Autodesk Inventor part; units mm, degrees
ref_plane "YZ Plane" through (0, 0, 0) normal (1, 0, 0) x (0, 1, 0)
ref_plane "XZ Plane" through (0, 0, 0) normal (0, 1, 0) x (-1, 0, 0)
ref_plane "XY Plane" through (0, 0, 0) normal (0, 0, 1) x (1, 0, 0)
sketch "Sketch1" plane through (0, 0, 0) normal (0, 0, 1) x (1, 0, 0)
  line L0 (0, 4) -> (0, 0)
  line L1 (0, 0) -> (125, 0)
  line L2 (125, 0) -> (125, 23.5)
  line L3 (57, 23.5) -> (0, 4)
  line L4 (81, 23.5) -> (81, 14.5)
  line L5 (81, 14.5) -> (92, 14.5)
  line L6 (92, 14.5) -> (92, 23.5)
  line L7 (125, 23.5) -> (92, 23.5)
  line L8 (81, 23.5) -> (57, 23.5)
  circle A0 centre (99.5, 19) radius 2.25
  circle A1 centre (119.5, 19) radius 2.25
  circle A2 centre (28.2, 6) radius 2.25
  circle A3 centre (28.2, 6) radius 4.5 construction
  point P0 (92, 19)
  dimension "d0" = 4
  dimension "d1" = 125
  dimension "d2" = 9
  dimension "d3" = 11
  dimension "d4" = 33
  dimension "d5" = 24
  dimension "d6" = 23.5
  dimension "d7" = 4.5
  dimension "d8" = 4.5
  dimension "d9" = 5.5
  dimension "d10" = 20
  dimension "d11" = 4.5
  dimension "d12" = 9
  dimension "d13" = 6
  dimension "d14" = 28.2
extrude "Extrusion1" add sketch "Sketch1" along normal blind 6.5
sketch "Sketch2" plane through (0, 0, 6.5) normal (0, 0, 1) x (1, 0, 0)
  line L0 (0, 0) -> (125, 0)
  line L1 (125, 23.5) -> (92, 23.5)
  line L2 (17, 0) -> (25, 0)
  line L3 (25, 0) -> (25, -4.5)
  line L4 (23, -6.5) -> (19, -6.5)
  line L5 (17, -4.5) -> (17, 0)
  line L6 (96, 0) -> (104, 0)
  line L7 (104, 0) -> (104, -19)
  line L8 (102, -21) -> (98, -21)
  line L9 (96, -19) -> (96, 0)
  line L10 (68, 0) -> (76, 0)
  line L11 (76, 0) -> (76, -19)
  line L12 (74, -21) -> (70, -21)
  line L13 (68, -19) -> (68, 0)
  line L14 (92, 23.5) -> (100, 23.5)
  line L15 (100, 23.5) -> (100, 29.5)
  line L16 (98, 31.5) -> (94, 31.5)
  line L17 (92, 29.5) -> (92, 23.5)
  arc A0 (17, -4.5) -> (19, -6.5) centre (19, -4.5) ccw
  arc A1 (23, -6.5) -> (25, -4.5) centre (23, -4.5) ccw
  arc A2 (96, -19) -> (98, -21) centre (98, -19) ccw
  arc A3 (102, -21) -> (104, -19) centre (102, -19) ccw
  arc A4 (68, -19) -> (70, -21) centre (70, -19) ccw
  arc A5 (74, -21) -> (76, -19) centre (74, -19) ccw
  arc A6 (94, 31.5) -> (92, 29.5) centre (94, 29.5) ccw
  arc A7 (100, 29.5) -> (98, 31.5) centre (98, 29.5) ccw
  line L18 (92, 23.5) -> (92, 14.5)
  dimension "d17" = 2
  dimension "d18" = 17
  dimension "d20" = 8
  dimension "d21" = 8
  dimension "d22" = 8
  dimension "d24" = 6.5
  dimension "d25" = 43
  dimension "d26" = 20
  dimension "d29" = 8
  dimension "d40" = 8
  dimension "d41" = 2
  dimension "d42" = 2
  dimension "d45" = 21
sketch "Sketch3" plane through (0, 0, 6.5) normal (0, 0, 1) x (1, 0, 0)
  circle A0 centre (119.5, 19) radius 2.25
  circle A1 centre (109.5, 19.599) radius 2.75
  circle A2 centre (86.5, 19.599) radius 7.5 construction
  dimension "d35" = 5.5
  dimension "d36" = 15
  dimension "d37" = 10
extrude "Extrusion3" cut sketch "Sketch3" against normal blind 6.5 contours A1
extrude "Extrusion4" add sketch "Sketch2" against normal blind 6.5
properties part number "x_motor_upper_nut_stop" material "Plywood, Finish"
Verification items for the finished model (mm, model axes). A direction names the side the tool comes from. Round coordinates to 2 decimals unless told otherwise and drop trailing zeros. Write each loop counter-clockwise with the first axis right and the second up, starting at its lowest first coordinate (ties: lowest second). Pieces come first, ordered by that corner, then holes.
1. Section check C-C on y = 25. Enter the section's corners in (x, z), plus the area to 3 significant figures.
2. Gauge pin test, flat ends, axial feed: P1, Ø3, axis at y = -13, z = 2.5, coming from the +X side; P2, Ø3.5, axis at y = -3, z = 2.5, coming from the -X side; P3, Ø3, axis at x = 116.5, z = 4.5, coming from the +Y side; P4, Ø2, axis at x = 97, z = 1, coming from the -Y side. Record the tip position at first contact, or that the pin passes through.
3. Section check A-A on x = 119.5. Enter the section's corners in (y, z).
4. Draft check along Y on faces 6 (the flat face through (104, -9, 3)), 7 (the cylindrical face through (107.318, 17.926, 3.296)), 8 (the flat face through (28.899, 13.887, 3.204)), 9 (the flat face through (21, -6.5, 3)). Enter one of: +Y half, -Y half, draft (parallel to the pull), parting line (faces both ways), or undercut.
5. Section check B-B on y = 6. Enter the section's corners in (x, z), plus the area to 3 significant figures.
6. Section check D-D on x = 62. Enter the section's corners in (y, z).
7. Access from +Z, -Z, +X, -X, +Y, -Y to the whole of each face (thin tool, end or side, straight path). Record for faces 1 (the flat face through (114, 0, 3)), 2 (the flat face through (100, 26, 3)), 3 (the flat face through (69, 23.5, 3)), 4 (the flat face through (25, -2, 3)), 5 (the flat face through (8, 0, 3)).
8. Scan lines: L1, parallel to X at y = -1.5, z = 4; L2, parallel to Y at x = 90, z = 6; L3, parallel to Y at x = 109.5, z = 3.25. Record each from-to range of solid material in increasing order.
Answer:
1. outline: (92, 0) - (100, 0) - (100, 6.5) - (92, 6.5) - close
1. area: 52.0 mm2
2. P1: stops at x = 104
2. P2: stops at x = 17
2. P3: stops at y = 23.5
2. P4: stops at y = -21
3. outline: (0, 0) - (16.75, 0) - (16.75, 6.5) - (0, 6.5) - close; (21.25, 0) - (23.5, 0) - (23.5, 6.5) - (21.25, 6.5) - close
4. face 6: draft
4. face 7: undercut
4. face 8: +Y half
4. face 9: -Y half
5. outline: (5.85, 0) - (25.95, 0) - (25.95, 6.5) - (5.85, 6.5) - close; (30.45, 0) - (125, 0) - (125, 6.5) - (30.45, 6.5) - close
5. area: 745 mm2
6. outline: (0, 0) - (23.5, 0) - (23.5, 6.5) - (0, 6.5) - close
7. face 1: +Z, -Z, +X, -Y
7. face 2: +Z, -Z, +X, +Y
7. face 3: +Z, -Z, -X, +Y
7. face 4: +Z, -Z, -Y
7. face 5: +Z, -Z, -X, -Y
8. L1: x = 17 to 25, 68 to 76, 96 to 104
8. L2: y = 0 to 14.5
8. L3: y = 0 to 16.85, 22.35 to 23.5
